```python
from build123d import *

# Parameters (mm, degrees)
RESSALTO_EXTRUS_O1_DEPTH = 4


with BuildPart() as part:
    # Esboço1 → Ressalto-extrusão1 (new body)
    with BuildSketch(Plane.XY):
        with BuildLine():
            Line((0.1, 0), (0.1, 0.8))
            Line((0.1, 0.8), (33.077498183, 0.8))
            Line((33.077498183, 0.8), (33.908082875, 0.8))
            ThreePointArc((33.908082875, 0.8), (35.05690323, -1.973497683), (32.283405548, -0.824677327))
            Line((32.283405548, -0.824677327), (32.083405548, -0.824677327))
            ThreePointArc((32.083405548, -0.824677327), (35.198324587, -2.114919039), (33.908082875, 1))
            Line((33.908082875, 1), (0, 1))
            ThreePointArc((0, 1), (-0.070710678, 0.970710678), (-0.1, 0.9))
            Line((-0.1, 0.9), (-0.1, 0.8))
            Line((-0.1, 0.8), (-0.1, 0))
            ThreePointArc((-0.1, 0), (0, -0.1), (0.1, 0))
        make_face()
    extrude(amount=RESSALTO_EXTRUS_O1_DEPTH)


solid = part.part
```
Geometry check sheet. Reference: the model listing, model coordinates, mm. Coordinates: 2 decimals unless noted, no trailing zeros. Order: outer loops, then holes, each group sorted by start corner. A loop starts at its lowest first (then second) coordinate and runs counter-clockwise, first axis right, second up.
Q1. Draft check along Y on faces 1 (the face through (17, 1, 2)), 2 (the face through (35.155, -2.157, 1.972)), 3 (the face through (35.094, -1.935, 1.972)). Enter one of: released by +Y, released by -Y, zero draft, split by the parting line, or undercut.
Reply:
face 1: released by +Y
face 2: split by the parting line
face 3: undercut
Q2. Sectioned sample at C-C on x = 12. Record the cut outline in (y, z).
Reply:
outline: (0.8, 0) - (1, 0) - (1, 4) - (0.8, 4) - close
Q3. Thickness scan on probe 1 along Y at (x, z) = (22, 1.8); probe 2 along X at (y, z) = (-2.25, 0.3); probe 3 along X at (y, z) = (-1, 1.05). Record the ranges inside material, lowest first.
Reply:
probe 1: y = 0.8 to 1
probe 2: x = 32.77 to 33.13, 34.69 to 35.05
probe 3: x = 32.09 to 32.29, 35.52 to 35.72
Q4. Depth check by flat-ended pin: pin 1 Ø2 at (x, z) = (13.5, 2) entering from -Y; pin 2 Ø0.6 at (y, z) = (0.5, 2.5) entering from +X; pin 3 Ø2 at (y, z) = (-0.5, 1) entering from -X. Enter the tip coordinate at first touch or a pass-through.
Reply:
pin 1: stops at y = 0.8
pin 2: stops at x = 35.42
pin 3: stops at x = -0.1
Q5. Sectioned sample at B-B on y = 0.3. Record the cut outline in (x, z).
Reply:
outline: (-0.1, 0) - (0.1, 0) - (0.1, 4) - (-0.1, 4) - close; (35.08, 0) - (35.34, 0) - (35.34, 4) - (35.08, 4) - close
Q6. Sectioned sample at A-A on z = 0.55. Record the cut outline in (x, y), and give its area (3 significant figures).
Reply:
outline: (-0.1, 0) arc R0.1 ccw to (0.1, 0) - (0.1, 0.8) - (33.91, 0.8) arc R1.62 cw (long way) to (32.28, -0.82) - (32.08, -0.82) arc R1.82 ccw (long way) to (33.91, 1) - (0, 1) arc R0.1 ccw to (-0.1, 0.9) - close
area: 8.60 mm2
